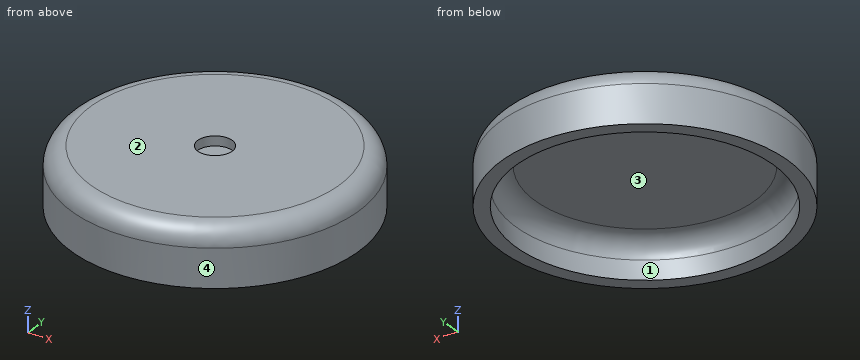
```python
from build123d import *

# Parameters (mm, degrees)
SKETCH1_R           = 15
BOSS_EXTRUDE1_DEPTH = 6
FILLET1_R           = 2
SKETCH2_R           = 13.5
CUT_EXTRUDE1_DEPTH  = 4
FILLET2_R           = 2
SKETCH4_R           = 1.8
CUT_EXTRUDE3_DEPTH  = 1


with BuildPart() as part:
    # Sketch1 → Boss-Extrude1 (new body)
    with BuildSketch(Plane.XY):
        Circle(SKETCH1_R)
    extrude(amount=BOSS_EXTRUDE1_DEPTH)

    # Fillet1
    fillet1_edges = [part.edges().sort_by_distance(p)[0] for p in [
        (-15, 0, 6),
    ]]
    fillet(fillet1_edges, radius=FILLET1_R)

    # Sketch2 → Cut-Extrude1 (cut)
    with BuildSketch(Plane(origin=(0, 0, 0), x_dir=(-1, 0, 0), z_dir=(0, 0, -1))):
        Circle(SKETCH2_R)
    extrude(amount=-CUT_EXTRUDE1_DEPTH, mode=Mode.SUBTRACT)

    # Fillet2
    fillet2_edges = [part.edges().sort_by_distance(p)[0] for p in [
        (13.5, 0, 4),
    ]]
    fillet(fillet2_edges, radius=FILLET2_R)

    # Sketch4 → Cut-Extrude3 (cut)
    with BuildSketch(Plane.XY.offset(6)):
        Circle(SKETCH4_R)
    extrude(amount=-CUT_EXTRUDE3_DEPTH, mode=Mode.SUBTRACT)


solid = part.part
```
Check sheet for the modelled part. Datum: model origin and axes. Units: mm. Face numbers are marked on the shaded views. Coordinates: 2 decimals unless noted, no trailing zeros. Order: outer loops, then holes, each group sorted by start corner. A loop starts at its lowest first (then second) coordinate and runs counter-clockwise, first axis right, second up. Notation, with made-up numbers: (-35.75, 11.5) -> (-27.75, 11.5) arc R37 ccw to (-27.75, 48.5) -> close; hole circle Ø11 at (-25.5, 25). An arc over 180 degrees is marked (long way). Write item = value, one per line. Start each with the question number.
1) Cross-section at A-A (y = 0). Enter the section's corners in (x, z), then the cut area to 3 significant figures.
2) Cross-section at C-C (z = 1.1). Enter the section's corners in (x, y), then the cut area to 3 significant figures.
3) Mould release check, pull along X, two halves, no side actions. Record for the marked faces 1, 2, 3 and 4: +X half, -X half, draft (parallel to the pull), parting line (faces both ways), or undercut.
4) Go/stop test with flat-tipped pins: P1, Ø2, axis at y = -6.5, z = 1.5, coming from the -X side; P2, Ø3, axis at y = -3, z = 5.5, coming from the +X side; P3, Ø3, axis at x = 0, y = 0, coming from the -Z side. Record where each tip stops, or that it passes through.
5) Cross-section at D-D (z = 2.95). Enter the section's corners in (x, y), then the cut area to 3 significant figures.
6) Material ranges on L1, parallel to Y at x = 0, z = 0.9; L2, parallel to Z at x = 1.5, y = 6.5; L3, parallel to X at y = 11.25, z = 1.7, recorded low to high.
Ans:
q1.outline = (-15, 0) -> (-13.5, 0) -> (-13.5, 2) arc R2 cw to (-11.5, 4) -> (11.5, 4) arc R2 cw to (13.5, 2) -> (13.5, 0) -> (15, 0) -> (15, 4) arc R2 ccw to (13, 6) -> (1.8, 6) -> (1.8, 5) -> (-1.8, 5) -> (-1.8, 6) -> (-13, 6) arc R2 ccw to (-15, 4) -> close
q1.area = 68.4 mm²
q2.outline = circle Ø30 at (0, 0); hole circle Ø27 at (0, 0)
q2.area = 134 mm²
q3.face_1 = undercut
q3.face_2 = draft
q3.face_3 = undercut
q3.face_4 = parting line
q4.P1 = -13.96
q4.P2 = 14.83
q4.P3 = 4
q5.outline = circle Ø30 at (0, 0); hole circle Ø26.52 at (0, 0)
q5.area = 154 mm²
q6.L1 = -15 to -13.5, 13.5 to 15
q6.L2 = 4 to 6
q6.L3 = -9.92 to -7.46, 7.46 to 9.92
